```python
from build123d import *

# Parameters (mm, degrees)
F2_W     = 25.146
F2_H     = 4.7498
F3_DEPTH = 34.6974
F4_R     = 0.381


with BuildPart() as f1:
    # F0 (on Right) → F1 (revolve)
    with BuildSketch(Plane.YZ):
        Polygon((-12.6492, 0.1524), (-12.6492, 34.6964), (-16.6624, 34.6964), (-16.6624, 31.6484), (-14.224, 31.6484), (-14.224, 12.8524), (-13.2842, 0.1524), align=None)
    revolve(axis=Axis((0, 0, 4.6482), (0, 0, -1)))

    # F2 (on Top) → F3 (cut, through all)
    with BuildSketch(Plane.XY):
        with Locations((-12.827, 0)):
            Rectangle(F2_W, F2_H)
    extrude(amount=F3_DEPTH, mode=Mode.SUBTRACT)

    # F4
    f4_edges = [f1.edges().sort_by_distance(p)[0] for p in [
        (-13.547512, -2.3749, 6.502381),
        (-14.024337, -2.3749, 22.2504),
        (-13.547512, 2.3749, 6.502381),
        (-14.024337, 2.3749, 22.2504),
        (-15.25831, -2.3749, 31.6484),
        (-15.25831, 2.3749, 31.6484),
    ]]
    fillet(f4_edges, radius=F4_R)


solid = f1.part
```
CAD build for the part. Positions are in the model's coordinates, mm. A direction names the side the tool comes from. Coordinates: 2 decimals unless noted, no trailing zeros. Write each loop counter-clockwise with the first axis right and the second up, starting at its lowest first coordinate (ties: lowest second). Pieces come first, ordered by that corner, then holes.
(1) 3-axis set-ups, long thin cutter, end or side, ignore diameter. For faces 1 (the face through (12.64, 0.52, 17.67)), 2 (the face through (-13, -2.375, 22)), 3 (the face through (14.21, 0.59, 22.12)): which of +Z, -Z, +X, -X, +Y, -Y reach the whole face in a straight line?
(2) Cut at A-A, the plane x = 0. List the corners of the cut face in (y, z).
(3) Flat gauge pins, fed straight in: pin 1 (1 mm diameter, centred on y = -1, z = 4, fed in from +X); pin 2 (4 mm diameter, centred on y = -2.5, z = 13, fed in from +X); pin 3 (4 mm diameter, centred on x = -4.5, z = 29.5, fed in from +Y); pin 4 (10 mm diameter, centred on x = -1.5, z = 28, fed in from +Y). Where does each tip first touch, or does it go through?
(4) Drill centre lines: probe 1 along Y at (x, z) = (0, 25); probe 2 along X at (y, z) = (0, 18); probe 3 along Z at (x, y) = (14.5, -5). Where is each one in solid material? Low to high.
(5) Cut at B-B, the plane y = 0. List the corners of the cut face in (x, z), and give its area (3 significant figures).
(6) Cut at C-C, the plane z = 18. List the corners of the cut face in (x, y), and give its area (3 significant figures).
Geometry says:
1. face 1: +Z, -Z
1. face 2: +Z, -Z, -X
1. face 3: -Z
2. outline: (-16.66, 31.65) - (-14.22, 31.65) - (-14.22, 12.85) - (-13.28, 0.15) - (-12.65, 0.15) - (-12.65, 34.7) - (-16.66, 34.7) - close; (12.65, 0.15) - (13.28, 0.15) - (14.22, 12.85) - (14.22, 31.65) - (16.66, 31.65) - (16.66, 34.7) - (12.65, 34.7) - close
3. pin 1: stops at x = 13.58
3. pin 2: stops at x = 14.22
3. pin 3: stops at y = 14
3. pin 4: stops at y = 16.66
4. probe 1: y = -14.22 to -12.65, 12.65 to 14.22
4. probe 2: x = 12.65 to 14.22
4. probe 3: z = 31.65 to 34.7
5. outline: (12.65, 0.15) - (13.28, 0.15) - (14.22, 12.85) - (14.22, 31.65) - (16.66, 31.65) - (16.66, 34.7) - (12.65, 34.7) - close
5. area: 55.9 mm2
6. outline: (-13.94, -2.83) arc R14.22 ccw (long way) to (-13.94, 2.83) arc R0.38 ccw to (-13.57, 2.37) - (-12.42, 2.37) arc R12.65 cw (long way) to (-12.42, -2.37) - (-13.57, -2.37) arc R0.38 ccw to start
6. area: 125 mm2
